Geometry: final body of the model. Coordinates: model frame, mm. Face numbers are marked on the shaded views. A direction names the side the tool comes from. Give positions to 0.01 mm unless a question says otherwise; leave off trailing zeros. Loops run counter-clockwise (first coordinate to the right, second up) from the corner with the lowest first, then second, coordinate; pieces in that order, holes last. Notation, with made-up numbers: M 20.5,35.25 L 32.5,35.25 A26 cw 32.5,65.25 Z; hole C 68,85.5 d10. An arc over 180 degrees is marked long. Put each result on its own line as item: value.
```python
from build123d import *

# Parameters (mm, degrees)
F0_W     = 78.2169550657
F0_H     = 84.6516340971
F1_DEPTH = 8.89
F2_DEPTH = 53.66258
F3_DEPTH = 65.51676
F4_T     = -1.27
F5_DEPTH = 25.4
F6_DEPTH = 25.4
F7_R     = 1.27


with BuildPart() as f1:
    # F0 (on Top) → F1 (new body)
    with BuildSketch(Plane.XY):
        with Locations((-39.1084775329, 34.8306708038)):
            Rectangle(F0_W, F0_H)
    extrude(amount=F1_DEPTH)

    # F2 (cut): a face of the model
    f2_faces = [f1.faces().sort_by_distance(p)[0] for p in [
        (-39.1084775329, -7.4951462448, 4.445),
    ]]
    extrude(f2_faces, amount=-F2_DEPTH, mode=Mode.SUBTRACT)

    # F3 (cut): a face of the model
    f3_faces = [f1.faces().sort_by_distance(p)[0] for p in [
        (0, 61.6619608038, 4.445),
    ]]
    extrude(f3_faces, amount=-F3_DEPTH, mode=Mode.SUBTRACT)

    # F4
    f4_openings = [f1.faces().sort_by_distance(p)[0] for p in [
        (-65.51676, 61.661961, 4.445),
    ]]
    offset(amount=F4_T, openings=f4_openings)

    # F5 (cut): a face of the model
    f5_faces = [f1.faces().sort_by_distance(p)[0] for p in [
        (-71.2318575329, 61.6619608038, 1.27),
    ]]
    extrude(f5_faces, amount=-F5_DEPTH, mode=Mode.SUBTRACT)

    # F6 (cut): a face of the model
    f6_faces = [f1.faces().sort_by_distance(p)[0] for p in [
        (-76.9469550657, 61.6619608038, 3.81),
    ]]
    extrude(f6_faces, amount=-F6_DEPTH, mode=Mode.SUBTRACT)

    # F7
    f7_edges = [f1.edges().sort_by_distance(p)[0] for p in [
        (-71.866858, 46.167434, 8.89),
        (-71.866858, 77.156488, 8.89),
    ]]
    fillet(f7_edges, radius=F7_R)


solid = f1.part
```
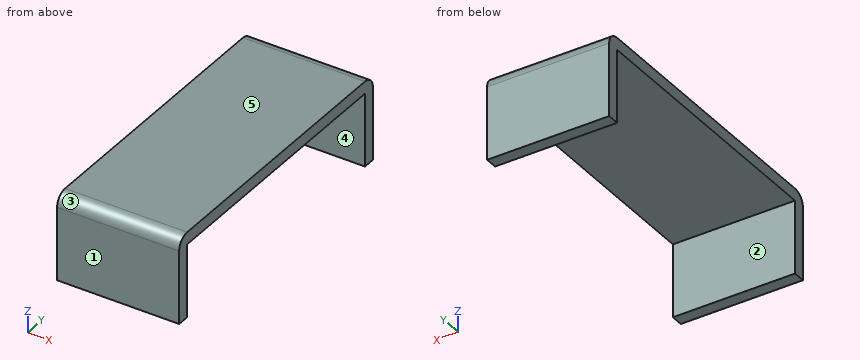
Item 1: Section C-C on y = 54. Output: boundary loops of the cut face in (x, z), then the cut area to 3 significant figures.
Output values:
outline: M -78.22,7.62 L -65.52,7.62 L -65.52,8.89 L -78.22,8.89 Z
area: 16.1 mm²
Item 2: Set-up query: the marked faces 1 and 2. Return all of +Z, -Z, +X, -X, +Y, -Y with unobstructed straight access to the full face (end or side cutting, diameter ignored); none if empty.
Output values:
face 1: +Z, -Z, +X, -X, -Y
face 2: -Z, +X, -X
Item 3: Section B-B on x = -71. Output: boundary loops of the cut face in (y, z), then the cut area to 3 significant figures.
Output values:
outline: M 46.17,0 L 47.44,0 L 47.44,7.62 L 75.89,7.62 L 75.89,0 L 77.16,0 L 77.16,7.62 A1.27 ccw 75.89,8.89 L 47.44,8.89 A1.27 ccw 46.17,7.62 Z
area: 58.0 mm²
Item 4: Mould query, pull axis Y, two halves, no side actions, for the marked faces 3, 4 and 5. Classes: pulls with the +Y half, pulls with the -Y half, needs draft (parallel to the pull), parting line crosses it, or undercut.
Output values:
face 3: pulls with the -Y half
face 4: undercut
face 5: needs draft
Item 5: Section A-A on z = 0.5. Output: boundary loops of the cut face in (x, y), then the cut area to 3 significant figures.
Output values:
outline: M -78.22,46.17 L -65.52,46.17 L -65.52,47.44 L -78.22,47.44 Z; M -78.22,75.89 L -65.52,75.89 L -65.52,77.16 L -78.22,77.16 Z
area: 32.3 mm²
Item 6: Line query: probe 1 along Y at (x, z) = (-71, 4); probe 2 along Z at (x, y) = (-76.25, 73.5). Output: solid intervals per line, ascending. Write a range as [from, to].
Output values:
probe 1: [46.17, 47.44], [75.89, 77.16]
probe 2: [7.62, 8.89]
Item 7: Pin query (flat end, axial travel): pin 1 Ø1 at (x, y) = (-73, 59.5) entering from -Z. Return the tip coordinate at first contact, or that it passes through.
Output values:
pin 1: z = 7.62
